from build123d import *

# Parameters (mm, degrees)
BOSS_EXTRUDE1_DEPTH      = 250
BOSS_EXTRUDE1_DEPTH_BACK = 250
SKETCH1_R                = 6
SKETCH1_R_2              = 5
BOSS_EXTRUDE2_START      = -25
SKETCH2_R                = 10
BOSS_EXTRUDE2_DEPTH      = 28
FILLET1_R                = 5
FILLET2_R                = 5


with BuildPart() as part:
    # Sketch1 → Boss-Extrude1 (new, two sides: drawn at the far end of the back side and taken through both)
    with BuildSketch(Plane.XY.offset(-BOSS_EXTRUDE1_DEPTH_BACK)):
        Circle(SKETCH1_R)
        Circle(SKETCH1_R_2, mode=Mode.SUBTRACT)
    extrude(amount=BOSS_EXTRUDE1_DEPTH + BOSS_EXTRUDE1_DEPTH_BACK)

    # Sketch2 → Boss-Extrude2 (add)
    with BuildSketch(Plane.XY.offset(250).offset(BOSS_EXTRUDE2_START)):
        Circle(SKETCH2_R)
    boss_extrude2 = extrude(amount=BOSS_EXTRUDE2_DEPTH)

    # Fillet1
    fillet1_edges = [part.edges().sort_by_distance(p)[0] for p in [
        (-10, 0, 253),
    ]]
    fillet(fillet1_edges, radius=FILLET1_R)

    # Mirror2: Boss-Extrude2 across plane
    add(boss_extrude2.mirror(Plane.XY))

    # Fillet2
    fillet2_edges = [part.edges().sort_by_distance(p)[0] for p in [
        (-10, 0, -253),
    ]]
    fillet(fillet2_edges, radius=FILLET2_R)


solid = part.part
CAD build for the part. Positions are in the model's coordinates, mm. A direction names the side the tool comes from. Give positions to 0.01 mm unless a question says otherwise; leave off trailing zeros. Order: outer loops, then holes, each group sorted by start corner. A loop starts at its lowest first (then second) coordinate and runs counter-clockwise, first axis right, second up. Notation, with made-up numbers: (82, 72.25) -> (124, 72.25) arc R20 cw to (124, 81.25) -> close; hole circle Ø4 at (84.25, -27.75). An arc over 180 degrees is marked (long way). Return JSON: item names as keys, results as strings.
Q1. Which spindle directions (+Z, -Z, +X, -X, +Y, -Y) get a long thin tool onto all of the face, cutting with end or side? Do faces 1 (the face through (-2.17, -9.76, 236.34)), 2 (the face through (0, -7, -225)). Say none if no direction does.
Working result:
{"face 1": "+Z, -Z", "face 2": "none"}
Q2. Mould opens along Z. For faces 3 (the face through (0, 0, 253)), 4 (the face through (-2.17, -9.76, -236.34)), 5 (the face through (0, 0, 225)) say: pulls with the +Z half, pulls with the -Z half, needs draft (parallel to the pull), parting line crosses it, or undercut.
Working result:
{"face 3": "pulls with the +Z half", "face 4": "needs draft", "face 5": "undercut"}
Q3. Drill centre lines: line 1 (Y direction, x = 0, z = 123); line 2 (Z direction, x = -2, y = 3). Where is each one in solid material? Low to high.
Working result:
{"line 1": "-6 to -5, 5 to 6", "line 2": "-253 to -225, 225 to 253"}
Q4. Saw through at A-A (z = -88.5). Write the cut outline in (x, y), then the cut area to 3 significant figures.
Working result:
{"outline": "circle Ø12 at (0, 0); hole circle Ø10 at (0, 0)", "area": "34.6 mm²"}
Q5. Flat gauge pins, fed straight in: pin 1 (4 mm diameter, centred on x = 5, y = -7.5, fed in from +Z); pin 2 (4 mm diameter, centred on x = -4, z = 126.5, fed in from +Y); pin 3 (12 mm diameter, centred on y = -1, z = -149, fed in from -X). Where does each tip first touch, or does it go through?
Working result:
{"pin 1": "z = 252.58", "pin 2": "y = 5.66", "pin 3": "x = -6"}
